from build123d import *

# Parameters (mm, degrees)
F0_R     = 21.1963
F1_DEPTH = 12.7
F2_R     = 3.7211
F3_DEPTH = 12.701
F4_T     = -1.778


with BuildPart() as f1:
    # F0 (on Front) → F1 (new body)
    with BuildSketch(Plane.XZ):
        Circle(F0_R)
    extrude(amount=F1_DEPTH)

    # F2 (on face) → F3 (cut, through all)
    with BuildSketch(Plane.XZ.offset(12.7)):
        Circle(F2_R)
    extrude(amount=-F3_DEPTH, mode=Mode.SUBTRACT)

    # F4
    f4_openings = [f1.faces().sort_by_distance(p)[0] for p in [
        (-20.596778, -12.7, 0),
    ]]
    offset(amount=F4_T, openings=f4_openings)


solid = f1.part
Geometry: final body of the model. Coordinates: model frame, mm. A direction names the side the tool comes from. Give positions to 0.01 mm unless a question says otherwise; leave off trailing zeros. Write each loop counter-clockwise with the first axis right and the second up, starting at its lowest first coordinate (ties: lowest second). Pieces come first, ordered by that corner, then holes.
(1) Cut plane A-A, the plane x = 0. Return loops of the section in (y, z).
(2) Cut plane D-D, the plane z = -14. Return loops of the section in (x, y).
(3) Ray query, line 1 (Z direction, x = 0, y = -8.75); line 2 (X direction, y = -7.5, z = 1.5); line 3 (X direction, y = -11.25, z = -4). Return the intervals inside material, ascending.
(4) First-contact query: P1, Ø2, axis at y = -8, z = -6, coming from the -X side; P2, Ø1, axis at x = -6, y = -10, coming from the -Z side; P3, Ø4, axis at x = -7.5, z = 1.5, coming from the -Y side. Flat tips, straight axial feed; report the tip coordinate or a pass-through.
(5) Access query for faces 1 (the cylindrical face through (-4.4, -7.3, -3.3)), 2 (the flat face through (19, -12.7, -6)). Directions: +Z, -Z, +X, -X, +Y, -Y. A direction counts if a zero-diameter tool reaches every point of the face in a straight line with its end or side. Return the directions, or none.
(6) Cut plane B-B, the plane y = -12. Return loops of the section in (x, z).
(7) Cut plane C-C, the plane z = 2.5. Return loops of the section in (x, y), then the cut area to 3 significant figures.
(8) Mould query, pull axis X, two halves, no side actions, for faces 3 (the flat face through (0, 0, -4)), 4 (the cylindrical face through (-4.595, -6.261, -20.692)), 5 (the flat face through (4, -1.778, -4)). Classes: released by +X, released by -X, zero draft, split by the parting line, or undercut.
Values follow:
1. outline: (-12.7, -21.2) - (0, -21.2) - (0, -3.72) - (-12.7, -3.72) - (-12.7, -5.5) - (-1.78, -5.5) - (-1.78, -19.42) - (-12.7, -19.42) - close; (-12.7, 3.72) - (0, 3.72) - (0, 21.2) - (-12.7, 21.2) - (-12.7, 19.42) - (-1.78, 19.42) - (-1.78, 5.5) - (-12.7, 5.5) - close
2. outline: (-15.91, -12.7) - (-13.46, -12.7) - (-13.46, -1.78) - (13.46, -1.78) - (13.46, -12.7) - (15.91, -12.7) - (15.91, 0) - (-15.91, 0) - close
3. line 1: z = -21.2 to -19.42, -5.5 to -3.72, 3.72 to 5.5, 19.42 to 21.2
3. line 2: x = -21.14 to -19.36, -5.29 to -3.41, 3.41 to 5.29, 19.36 to 21.14
3. line 3: x = -20.82 to -19, -3.77 to 3.77, 19 to 20.82
4. P1: stops at x = -20.6
4. P2: stops at z = -20.47
4. P3: stops at y = -1.78
5. face 1: -Y
5. face 2: +Z, -Z, +X, -X, -Y
6. outline: circle Ø42.39 at (0, 0); circle Ø11 at (0, 0); hole circle Ø38.84 at (0, 0); hole circle Ø7.44 at (0, 0)
7. outline: (-21.05, -12.7) - (-19.26, -12.7) - (-19.26, -1.78) - (-4.9, -1.78) - (-4.9, -12.7) - (-2.76, -12.7) - (-2.76, 0) - (-21.05, 0) - close; (2.76, -12.7) - (4.9, -12.7) - (4.9, -1.78) - (19.26, -1.78) - (19.26, -12.7) - (21.05, -12.7) - (21.05, 0) - (2.76, 0) - close
7. area: 151 mm2
8. face 3: zero draft
8. face 4: split by the parting line
8. face 5: undercut
